Check sheet for the modelled part. Datum: model origin and axes. Units: mm. Coordinates: 2 decimals unless noted, no trailing zeros. Loops run counter-clockwise (first coordinate to the right, second up) from the corner with the lowest first, then second, coordinate; pieces in that order, holes last.
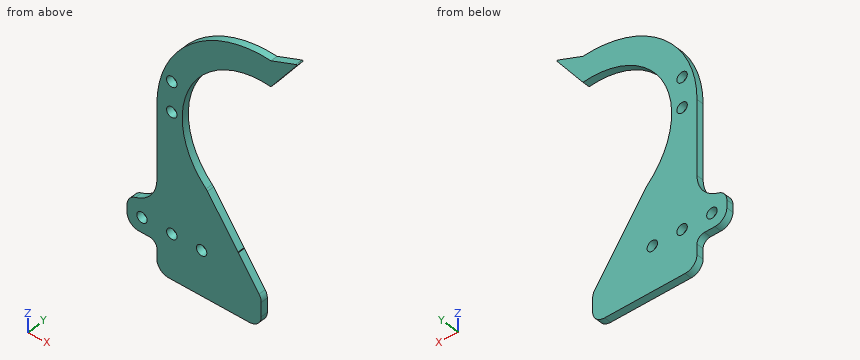
Autodesk Inventor part; units mm, degrees
ref_plane "YZ Plane" through (0, 0, 0) normal (1, 0, 0) x (0, 1, 0)
ref_plane "XZ Plane" through (0, 0, 0) normal (0, 1, 0) x (-1, 0, 0)
ref_plane "XY Plane" through (0, 0, 0) normal (0, 0, 1) x (1, 0, 0)
sketch "Sketch1" plane through (0, 0, 0) normal (0, 1, 0) x (-1, 0, 0)
  circle A0 centre (0, 0) radius 33.655
  circle A1 centre (0, 0) radius 44.45
  line L0 (0, 44.45) -> (0, 33.655)
  line L1 (7.4782, -32.8136) -> (9.9419, -43.3239)
  line L2 (0, -44.45) -> (44.45, 0)
  line L3 (0, -44.45) -> (0, -69.85)
  line L4 (0, -69.85) -> (38.1, -69.85) construction
  line L5 (-4.1275, 44.258) -> (-4.1275, 33.4009)
  line L6 (-4.1275, 44.258) -> (-15.6469, 48.7936)
  line L7 (-15.6469, 48.7936) -> (-4.1275, 33.4009)
  line L8 (0, -69.85) -> (44.45, -69.85)
  line L9 (44.45, -69.85) -> (44.45, 0)
  line L10 (44.45, -69.85) -> (69.85, -69.85)
  line L11 (69.85, -69.85) -> (69.85, -44.45)
  line L12 (69.85, -44.45) -> (44.45, -44.45)
  line L13 (69.85, -44.45) -> (69.85, -50.8)
  line L14 (69.85, -50.8) -> (63.5, -50.8)
  circle A2 centre (63.5, -50.8) radius 2.2225
  line L15 (63.5, -50.8) -> (50.8, -50.8)
  circle A3 centre (50.8, -50.8) radius 2.2225
  line L16 (50.8, -50.8) -> (50.8, -63.5)
  circle A4 centre (50.8, -63.5) radius 2.2225
  line L17 (50.8, -63.5) -> (63.5, -63.5)
  circle A5 centre (63.5, -63.5) radius 2.2225
  line L18 (44.45, 0) -> (38.1, 0)
  circle A6 centre (38.1, 0) radius 2.2225
  line L19 (38.1, 0) -> (38.1, 12.7)
  circle A7 centre (38.1, 12.7) radius 2.2225
  line L20 (57.15, -69.85) -> (57.15, -44.45)
  line L21 (0, -57.15) -> (30.7326, -13.7174)
  line L22 (0, -57.15) -> (69.85, -57.15)
  line L23 (50.8, -50.8) -> (38.1, -50.8)
  circle A8 centre (38.1, -50.8) radius 2.2225
  line L24 (38.1, -50.8) -> (25.4, -50.8)
  circle A9 centre (25.4, -50.8) radius 2.2225
  point P0 (13.7174, -30.7326)
  point P1 (30.7326, -13.7174)
  point P2 (-11.3028, 42.9889)
  point P3 (23.1613, -24.4175)
  point P4 (9.9025, -43.1554)
  point P5 (9.7529, -43.3669)
  point P6 (57.15, -57.15)
  point P7 (44.45, -57.15)
  dimension "d0" = 67.31
  dimension "d1" = 88.9
  dimension "d23" = 44.45
  dimension "d24" = 6.35
  dimension "d25" = 6.35
  dimension "d26" = 4.445
  dimension "d27" = 12.7
  dimension "d28" = 4.445
  dimension "d29" = 12.7
  dimension "d30" = 4.445
  dimension "d31" = 12.7
  dimension "d32" = 4.445
  dimension "d35" = 6.35
  dimension "d36" = 4.445
  dimension "d37" = 12.7
  dimension "d38" = 4.445
  dimension "d47" = 12.7
  dimension "d48" = 4.445
  dimension "d49" = 12.7
  dimension "d50" = 4.445
extrude "Extrusion1" add sketch "Sketch1" along normal blind 3 contours A0 L0 A1 L2 | A0 L5 A1 L0 | L2 A1 L1 L21 A0 | L7 A1 L5 | L9 L22 L21 A1 | A1 L7 L6 | L12 L20 L15 A3 L23 L9 | L23 A3 L16 L22 L9 | L22 L9 L8 L3 | L20 L22 L16 A3 L15
sketch "Sketch3" plane through (0, 3, 0) normal (0, 1, 0) x (1, 0, 0)
  point P0 (0, 0)
fillet "Fillet3" radius 0.254 1 edges at (15.6469, 1.5, 48.7936)
fillet "Fillet5" radius 12.7 1 edges at (-44.45, 1.5, -44.45)
sketch "Sketch4" plane through (0, 3, 0) normal (0, 1, 0) x (1, 0, 0)
  point P0 (0, 0)
fillet "Fillet9" radius 5.08 1 edges at (0, 1.5, -69.85)
fillet "Fillet10" radius 5.08 1 edges at (0, 1.5, -57.15)
fillet "Fillet11" radius 5.08 1 edges at (-23.1613, 1.5, -24.4175)
fillet "Fillet12" radius 5.08 2 edges at (-57.1495, 1.5, -44.45) (-57.15, 1.5, -44.45)
fillet "Fillet14" radius 5.08 1 edges at (-57.15, 1.5, -57.15)
fillet "Fillet15" radius 5.08 1 edges at (-44.45, 1.5, -69.85)
fillet "Fillet16" radius 3.175 1 edges at (-44.45, 1.5, -57.15)
properties part number "Climb hook_3DPrint"
1) Section check C-C on z = 12.7. Enter the section's corners in (x, y), plus the area to 3 significant figures.
Answer sheet:
outline: (-42.6, 0) - (-40.32, 0) - (-40.32, 3) - (-42.6, 3) - close; (-35.88, 0) - (-31.17, 0) - (-31.17, 3) - (-35.88, 3) - close
area: 21.0 mm2
2) Section check B-B on x = -13.5. Enter the section's corners in (y, z).
Answer sheet:
outline: (0, -69.85) - (3, -69.85) - (3, -38.07) - (0, -38.07) - close; (0, 30.83) - (3, 30.83) - (3, 42.35) - (0, 42.35) - close
3) Section check A-A on x = -25.4. Enter the section's corners in (y, z).
Answer sheet:
outline: (0, -69.85) - (3, -69.85) - (3, -53.02) - (0, -53.02) - close; (0, -48.58) - (3, -48.58) - (3, -22.08) - (0, -22.08) - close; (0, 22.08) - (3, 22.08) - (3, 36.48) - (0, 36.48) - close
4) Section check D-D on z = -50.8. Enter the section's corners in (x, y).
Answer sheet:
outline: (-57.15, 0) - (-53.02, 0) - (-53.02, 3) - (-57.15, 3) - close; (-48.58, 0) - (-40.32, 0) - (-40.32, 3) - (-48.58, 3) - close; (-35.88, 0) - (-27.62, 0) - (-27.62, 3) - (-35.88, 3) - close; (-23.18, 0) - (-4.49, 0) - (-4.49, 3) - (-23.18, 3) - close
5) Scan lines: line 1 (Z direction, x = -38.1, y = 2); line 2 (Z direction, x = -38, y = 0.45); line 3 (Z direction, x = -25.4, y = 2.3). Record each from-to range of solid material in increasing order.
Answer sheet:
line 1: z = -69.85 to -53.02, -48.58 to -2.22, 2.22 to 10.48, 14.92 to 22.9
line 2: z = -69.85 to -53.02, -48.58 to -2.22, 2.22 to 10.48, 14.92 to 23.06
line 3: z = -69.85 to -53.02, -48.58 to -22.08, 22.08 to 36.48
